```python
from build123d import *

# Parameters (mm, degrees)
F0_W          = 45
F0_H          = 35.2
F1_DEPTH      = 45
F2_W          = 29
F2_H          = 29
F3_DEPTH      = 22.5
F4_W          = 47
F4_H          = 47
F5_DEPTH      = 15.5
F6_W          = 47
F6_H          = 47
F7_DEPTH      = 28
F8_W          = 15
F8_H          = 15
F9_DEPTH      = 24.7
F9_DEPTH_BACK = 9
F11_START     = 7.5
F11_DEPTH     = 8
F13_START     = 7.5
F13_DEPTH     = 1.6
F15_START     = 4.7
F15_DEPTH     = 2.8
F17_START     = 4.7
F16_W         = 19
F16_H         = 19
F17_DEPTH     = 2.6
F18_R         = 1.5


with BuildPart() as f1:
    # F0 (on Right) → F1 (new body)
    with BuildSketch(Plane.YZ):
        Rectangle(F0_W, F0_H)
    extrude(amount=F1_DEPTH)

    # F2 (on Top) → F3 (cut, symmetric)
    with BuildSketch(Plane.XY):
        with Locations((14.5, 8)):
            Rectangle(F2_W, F2_H)
    extrude(amount=F3_DEPTH, both=True, mode=Mode.SUBTRACT)

    # F4 (on Top) → F5 (cut, symmetric)
    with BuildSketch(Plane.XY):
        with Locations((19.5, 3)):
            Rectangle(F4_W, F4_H)
    extrude(amount=F5_DEPTH, both=True, mode=Mode.SUBTRACT)

    # F6 (on Top) → F7 (cut)
    with BuildSketch(Plane.XY):
        with Locations((17.5, 5)):
            Rectangle(F6_W, F6_H)
    extrude(amount=-F7_DEPTH, mode=Mode.SUBTRACT)

    # F8 (on Top) → F9 (cut, two sides)
    with BuildSketch(Plane.XY) as f9_sk:
        with Locations((45, -22.5)):
            Rectangle(F8_W, F8_H)
    extrude(amount=-F9_DEPTH, mode=Mode.SUBTRACT)
    extrude(f9_sk.sketch, amount=F9_DEPTH_BACK, mode=Mode.SUBTRACT)

    # F10 (on Top) → F11 (join)
    with BuildSketch(Plane.XY.offset(F11_START)):
        Polygon((31, 22.5), (29, 22.5), (29, -6.5), (0, -6.5), (0, -8.5), (31, -8.5), align=None)
    extrude(amount=F11_DEPTH)

    # F12 (on Top) → F13 (join)
    with BuildSketch(Plane.XY.offset(F13_START)):
        Polygon((29, -6.5), (29, 22.5), (19, 22.5), (19, 3.5), (0, 3.5), (0, -6.5), align=None)
    extrude(amount=F13_DEPTH)

    # F14 (on Top) → F15 (join)
    with BuildSketch(Plane.XY.offset(F15_START)):
        Polygon((21, 22.5), (19, 22.5), (19, 3.5), (0, 3.5), (0, 1.5), (21, 1.5), align=None)
    extrude(amount=F15_DEPTH)

    # F16 (on Top) → F17 (join)
    with BuildSketch(Plane.XY.offset(F17_START)):
        with Locations((9.5, 13)):
            Rectangle(F16_W, F16_H)
    extrude(amount=F17_DEPTH)

    # F18
    f18_edges = [f1.edges().sort_by_distance(p)[0] for p in [
        (22.5, -22.5, 17.6),
        (45, 0, 17.6),
        (45, 3.75, -17.6),
        (18.75, -22.5, -17.6),
        (14.5, -6.5, 17.6),
        (29, 8, 17.6),
        (29, -6.5, 13.35),
        (45, -22.5, 13.3),
        (29, 8, 9.1),
        (14.5, -6.5, 9.1),
        (19, 13, 9.1),
        (9.5, 3.5, 9.1),
        (19, 3.5, 8.2),
        (31, 7, 7.5),
        (21, 12, 4.7),
        (10.5, 1.5, 4.7),
        (15.5, -8.5, 7.5),
        (21, 1.5, 6.1),
        (31, -8.5, 11.5),
    ]]
    fillet(f18_edges, radius=F18_R)


solid = f1.part
```
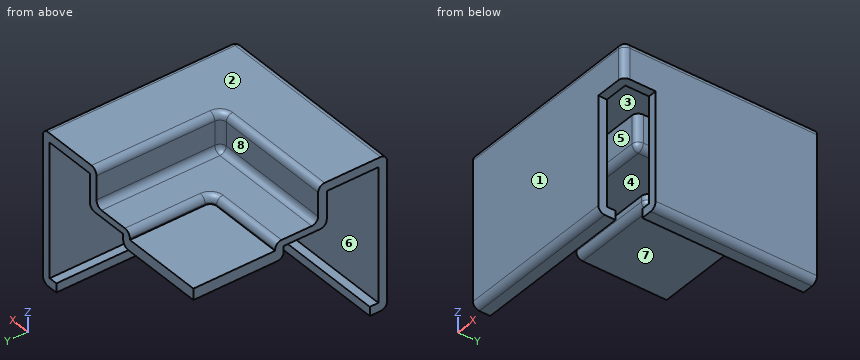
Check sheet for the modelled part. Datum: model origin and axes. Units: mm. Face numbers are marked on the shaded views. A direction names the side the tool comes from. Give positions to 0.01 mm unless a question says otherwise; leave off trailing zeros. Order: outer loops, then holes, each group sorted by start corner. A loop starts at its lowest first (then second) coordinate and runs counter-clockwise, first axis right, second up. Notation, with made-up numbers: (53.5, 65) -> (102.5, 65) arc R10 ccw to (102.5, 72) -> close; hole circle Ø1 at (19.25, 83.5). An arc over 180 degrees is marked (long way). Return JSON: item names as keys, results as strings.
1. Mould release check, pull along Y, two halves, no side actions. Record for the marked faces 1, 2 and 3: +Y half, -Y half, draft (parallel to the pull), parting line (faces both ways), or undercut.
From the geometry:
{"face 1": "-Y half", "face 2": "draft", "face 3": "undercut"}
2. Cross-section at A-A, the plane z = -3.5. Record the cut outline in (x, y), plus the area to 3 significant figures.
From the geometry:
{"outline": "(0, -22.5) -> (37.5, -22.5) -> (37.5, -20.5) -> (0, -20.5) -> close; (43, -15) -> (45, -15) -> (45, 22.5) -> (43, 22.5) -> close", "area": "150 mm^2"}
3. Cross-section at C-C, the plane y = 19. Record the cut outline in (x, z).
From the geometry:
{"outline": "(0, 4.7) -> (19.5, 4.7) arc R1.5 ccw to (21, 6.2) -> (21, 7.5) -> (29.5, 7.5) arc R1.5 ccw to (31, 9) -> (31, 15.5) -> (43, 15.5) -> (43, -15.5) -> (41, -15.5) -> (41, -17.6) -> (43.5, -17.6) arc R1.5 ccw to (45, -16.1) -> (45, 16.1) arc R1.5 ccw to (43.5, 17.6) -> (30.5, 17.6) arc R1.5 ccw to (29, 16.1) -> (29, 10.6) arc R1.5 cw to (27.5, 9.1) -> (20.5, 9.1) arc R1.5 ccw to (19, 7.6) -> (19, 7.3) -> (0, 7.3) -> close"}
4. Go/stop test with flat-tipped pins: P1, Ø0.6, axis at x = 11, z = -17, coming from the +Y side; P2, Ø4.5, axis at y = 2, z = 13.5, coming from the -X side; P3, Ø1.1, axis at y = 11.5, z = -16.5, coming from the -X side. Record where each tip stops, or that it passes through.
From the geometry:
{"P1": "y = -18.5", "P2": "x = 29", "P3": "x = 41"}
5. Cross-section at D-D, the plane x = 32.5. Record the cut outline in (y, z).
From the geometry:
{"outline": "(-22.5, -16.1) arc R1.5 ccw to (-21, -17.6) -> (-18.5, -17.6) -> (-18.5, -15.5) -> (-20.5, -15.5) -> (-20.5, 15.5) -> (22.5, 15.5) -> (22.5, 17.6) -> (-21, 17.6) arc R1.5 ccw to (-22.5, 16.1) -> close"}
6. Material ranges on probe 1 along Z at (x, y) = (2, -19.5); probe 2 along Y at (x, z) = (26, 9); probe 3 along Y at (x, z) = (7.5, 13), recorded low to high. Write a range as [from, to].
From the geometry:
{"probe 1": "[-17.6, -15.5], [15.5, 17.6]", "probe 2": "[-22.5, -20.5], [-8.5, 22.5]", "probe 3": "[-22.5, -20.5], [-8.5, -6.5]"}
7. Cross-section at B-B, the plane x = 4. Record the cut outline in (y, z), plus the area to 3 significant figures.
From the geometry:
{"outline": "(-22.5, -16.1) arc R1.5 ccw to (-21, -17.6) -> (-18.5, -17.6) -> (-18.5, -15.5) -> (-20.5, -15.5) -> (-20.5, 15.5) -> (-8.5, 15.5) -> (-8.5, 9) arc R1.5 ccw to (-7, 7.5) -> (1.5, 7.5) -> (1.5, 6.2) arc R1.5 ccw to (3, 4.7) -> (22.5, 4.7) -> (22.5, 7.3) -> (3.5, 7.3) -> (3.5, 7.6) arc R1.5 ccw to (2, 9.1) -> (-5, 9.1) arc R1.5 cw to (-6.5, 10.6) -> (-6.5, 16.1) arc R1.5 ccw to (-8, 17.6) -> (-21, 17.6) arc R1.5 ccw to (-22.5, 16.1) -> close", "area": "189 mm^2"}
8. Set-up check for the marked faces 4, 5, 6, 7 and 8: record each of +Z, -Z, +X, -X, +Y, -Y from which the full face is reachable in a straight line by a thin tool's end or side.
From the geometry:
{"face 4": "-Z", "face 5": "-Z, -X", "face 6": "-X", "face 7": "-Z, -X, +Y", "face 8": "+Z, -X, +Y"}
